Source: CAD feature listing. Evaluate the final solid. Frame: model axes, mm. A direction names the side the tool comes from. Give positions to 0.01 mm unless a question says otherwise; leave off trailing zeros. Order: outer loops, then holes, each group sorted by start corner. A loop starts at its lowest first (then second) coordinate and runs counter-clockwise, first axis right, second up. Notation, with made-up numbers: (-29, 85) -> (-20, 85) arc R6 ccw to (-20, 89) -> close; hole circle Ø6 at (-16, -11). An arc over 180 degrees is marked (long way). Answer in a Markdown table with one row per item.
```python
from build123d import *

# Parameters (mm, degrees)
SKETCH1_R           = 77.4600051
BOSS_EXTRUDE1_DEPTH = 3.175
SKETCH20_R          = 22.86
SKETCH20_R_2        = 2.0193
CUT_EXTRUDE10_DEPTH = 251.865681086
SKETCH21_R          = 2.0193
CUT_EXTRUDE11_DEPTH = 251.865681086
CUT_EXTRUDE12_DEPTH = 251.865681086
SKETCH23_R          = 2.54
CUT_EXTRUDE13_DEPTH = 3.175


with BuildPart() as part:
    # Sketch1 → Boss-Extrude1 (new body)
    with BuildSketch(Plane(origin=(0, 0, 0), x_dir=(1, 0, 0), z_dir=(0, 1, 0))):
        with Locations(Location((0, 0, 0), (0, 0, 270))):
            Circle(SKETCH1_R)
    extrude(amount=BOSS_EXTRUDE1_DEPTH)

    # Sketch20 → Cut-Extrude10 (cut, through all)
    with BuildSketch(Plane(origin=(-73.768816189, 25.4, -121.080352405), x_dir=(1, 0, 0), z_dir=(0, 1, 0))):
        with Locations(Location((73.768816189, -121.080352405, 0), (0, 0, 270))):
            Circle(SKETCH20_R)
        with Locations(Location((73.768816189, -88.060352405, 0), (0, 0, 270))):
            Circle(SKETCH20_R_2)
        with Locations(Location((106.788816189, -121.080352405, 0), (0, 0, 270))):
            Circle(SKETCH20_R_2)
        with Locations(Location((73.768816189, -154.100352405, 0), (0, 0, 270))):
            Circle(SKETCH20_R_2)
        with Locations(Location((40.748816189, -121.080352405, 0), (0, 0, 270))):
            Circle(SKETCH20_R_2)
    extrude(amount=-CUT_EXTRUDE10_DEPTH, mode=Mode.SUBTRACT)

    # Sketch21 → Cut-Extrude11 (cut, through all)
    with BuildSketch(Plane(origin=(-73.768816189, 25.4, -121.080352405), x_dir=(1, 0, 0), z_dir=(0, 1, 0))):
        with Locations(Location((48.605023435, -95.916559651, 0), (0, 0, 270))):
            Circle(SKETCH21_R)
    extrude(amount=-CUT_EXTRUDE11_DEPTH, mode=Mode.SUBTRACT)

    # Sketch22 → Cut-Extrude12 (cut, through all)
    with BuildSketch(Plane(origin=(-73.768816189, 25.4, -121.080352405), x_dir=(1, 0, 0), z_dir=(0, 1, 0))):
        with BuildLine():
            ThreePointArc((34.405967979, -136.122213123), (36.00963526, -139.786919397), (37.953573181, -143.283049568))
            ThreePointArc((37.953573181, -143.283049568), (46.974494303, -145.399596657), (49.091041391, -136.378675534))
            ThreePointArc((49.091041391, -136.378675534), (47.751609959, -133.969737166), (46.646635186, -131.444644817))
            ThreePointArc((46.646635186, -131.444644817), (38.18751743, -127.663095366), (34.405967979, -136.122213123))
        make_face()
    extrude(amount=-CUT_EXTRUDE12_DEPTH, mode=Mode.SUBTRACT)

    # Sketch23 → Cut-Extrude13 (cut)
    with BuildSketch(Plane(origin=(-73.768816189, 0, -121.080352405), x_dir=(1, 0, 0), z_dir=(0, -1, 0))):
        with Locations(Location((43.216869762, 151.632298832, 0), (0, 0, 270))):
            Circle(SKETCH23_R)
    extrude(amount=-CUT_EXTRUDE13_DEPTH, mode=Mode.SUBTRACT)


solid = part.part
```
(1) Section query D-D (x = 33.02). Return the cut outline in (y, z) (3 decimals).
A:
| item | result |
|---|---|
| outline | (0, -70.069) -> (3.175, -70.069) -> (3.175, -2.019) -> (0, -2.019) -> close; (0, 2.019) -> (3.175, 2.019) -> (3.175, 70.069) -> (0, 70.069) -> close |
(2) Access query for faces 4 (the flat face through (18, 0, 16)), 5 (the cylindrical face through (-37.78, 1.61, 18.66)). Directions: +Z, -Z, +X, -X, +Y, -Y. A direction counts if a zero-diameter tool reaches every point of the face in a straight line with its end or side. Return the directions, or none.
A:
| item | result |
|---|---|
| face 4 | +Z, -Z, +X, -X, -Y |
| face 5 | +Y, -Y |
(3) Section query C-C (y = 0.7). Give the number of separate pieces and of enclosed holes in the cut face, plus the area to 3 significant figures.
A:
| item | result |
|---|---|
| separate pieces | 1 |
| enclosed holes | 8 |
| area | 16,900 mm^2 |
(4) First-contact query: pin 1 Ø2.5 at (x, z) = (-25.16, -25.16) entering from +Y; pin 2 Ø1.5 at (x, y) = (-40.5, 0.5) entering from +Z. Flat tips, straight axial feed; report the tip coordinate or a pass-through.
A:
| item | result |
|---|---|
| pin 1 | passes through |
| pin 2 | stops at z = 66.48 |
(5) Pull-direction query (Z, two-part tool) for faces 1 (the cylindrical face through (23.27, 1.57, 73.88)), 2 (the cylindrical face through (-25.08, 1.61, -27.18)), 3 (the flat face through (18, 3.175, 16)); classes: +Z half, -Z half, draft (parallel to the pull), parting line (faces both ways), or undercut.
A:
| item | result |
|---|---|
| face 1 | parting line |
| face 2 | undercut |
| face 3 | draft |
(6) Section query B-B (z = -12). Return the cut outline in (x, y) (3 decimals).
A:
| item | result |
|---|---|
| outline | (-76.525, 0) -> (-19.457, 0) -> (-19.457, 3.175) -> (-76.525, 3.175) -> close; (19.457, 0) -> (76.525, 0) -> (76.525, 3.175) -> (19.457, 3.175) -> close |
(7) Ray query, probe 1 along X at (y, z) = (1.5, 0); probe 2 along X at (y, z) = (1.1, -11); probe 3 along X at (y, z) = (1.35, -33.5). Return the intervals inside material, ascending.
A:
| item | result |
|---|---|
| probe 1 | x = -77.46 to -35.04, -31 to -22.86, 22.86 to 31, 35.04 to 77.46 |
| probe 2 | x = -76.67 to -20.04, 20.04 to 76.67 |
| probe 3 | x = -69.84 to -1.96, 1.96 to 69.84 |
(8) Section query A-A (x = 0). Return the cut outline in (y, z) (3 decimals).
A:
| item | result |
|---|---|
| outline | (0, -77.46) -> (3.175, -77.46) -> (3.175, -35.039) -> (0, -35.039) -> close; (0, -31.001) -> (3.175, -31.001) -> (3.175, -22.86) -> (0, -22.86) -> close; (0, 22.86) -> (3.175, 22.86) -> (3.175, 31.001) -> (0, 31.001) -> close; (0, 35.039) -> (3.175, 35.039) -> (3.175, 77.46) -> (0, 77.46) -> close |
